```python
from build123d import *

# Parameters (mm, degrees)
F1_DEPTH = 30
F2_W     = 56
F2_H     = 56
F3_DEPTH = 100.001
F4_W     = 50
F4_H     = 15
F5_DEPTH = 60
F6_W     = 50
F6_H     = 15
F7_DEPTH = 30
F8_W     = 80
F8_H     = 80
F9_DEPTH = 2
F10_R    = 1
F11_R    = 1
F12_R    = 1
F13_R    = 1
F14_R    = 0.5
F15_R    = 0.5
F16_R    = 0.5


with BuildPart() as f1:
    # F0 (on Front) → F1 (new body, symmetric)
    with BuildSketch(Plane.XZ):
        Polygon((30, 49.2234811187), (0, 49.2234811187), (-30, 49.2234811187), (-30, -50.7765188813), (0, -21.0795458406), (30, -50.7765188813), align=None)
    extrude(amount=F1_DEPTH, both=True)

    # F2 (on face) → F3 (cut, through all)
    with BuildSketch(Plane.XY.offset(49.2234811187)):
        with Locations((-2.794e-06, 0)):
            Rectangle(F2_W, F2_H)
    extrude(amount=-F3_DEPTH, mode=Mode.SUBTRACT)

    # F4 (on face) → F5 (cut)
    with BuildSketch(Plane.XZ.offset(30)):
        with Locations((0, 38.2234811187)):
            Rectangle(F4_W, F4_H)
    extrude(amount=-F5_DEPTH, mode=Mode.SUBTRACT)

    # F6 (on Right) → F7 (cut, symmetric)
    with BuildSketch(Plane.YZ):
        with Locations((0, 38.2234811187)):
            Rectangle(F6_W, F6_H)
    extrude(amount=F7_DEPTH, both=True, mode=Mode.SUBTRACT)

    # F8 (on face) → F9 (join)
    with BuildSketch(Plane.XY.offset(49.2234811187)):
        Rectangle(F8_W, F8_H)
    extrude(amount=-F9_DEPTH)

    # F10
    f10_edges = [f1.edges().sort_by_distance(p)[0] for p in [
        (-29.000001, 25, 30.723481),
        (-29.000001, -25, 30.723481),
        (-29.000001, -25, 45.723481),
        (-29.000001, 25, 45.723481),
    ]]
    fillet(f10_edges, radius=F10_R)

    # F11
    f11_edges = [f1.edges().sort_by_distance(p)[0] for p in [
        (-25, 29, 45.723481),
        (-25, 29, 30.723481),
        (25, 29, 30.723481),
        (25, 29, 45.723481),
    ]]
    fillet(f11_edges, radius=F11_R)

    # F12
    f12_edges = [f1.edges().sort_by_distance(p)[0] for p in [
        (28.999999, 25, 45.723481),
        (28.999999, -25, 45.723481),
        (28.999999, -25, 30.723481),
        (28.999999, 25, 30.723481),
    ]]
    fillet(f12_edges, radius=F12_R)

    # F13
    f13_edges = [f1.edges().sort_by_distance(p)[0] for p in [
        (25, -29, 30.723481),
        (25, -29, 45.723481),
        (-25, -29, 45.723481),
        (-25, -29, 30.723481),
    ]]
    fillet(f13_edges, radius=F13_R)

    # F14
    f14_edges = [f1.edges().sort_by_distance(p)[0] for p in [
        (30, 30, -1.776519),
        (30, -30, -1.776519),
        (-30, 30, -1.776519),
        (-30, -30, -1.776519),
    ]]
    fillet(f14_edges, radius=F14_R)

    # F15
    f15_edges = [f1.edges().sort_by_distance(p)[0] for p in [
        (40, -40, 48.223481),
        (40, 0, 49.223481),
        (40, 0, 47.223481),
        (0, -40, 47.223481),
        (0, -40, 49.223481),
        (-40, -40, 48.223481),
        (-40, 0, 47.223481),
        (-40, 0, 49.223481),
        (0, 40, 47.223481),
        (0, 40, 49.223481),
        (-40, 40, 48.223481),
        (40, 40, 48.223481),
    ]]
    fillet(f15_edges, radius=F15_R)

    # F16
    f16_edges = [f1.edges().sort_by_distance(p)[0] for p in [
        (0, 30, 47.223481),
    ]]
    fillet(f16_edges, radius=F16_R)


solid = f1.part
```
Here's how the part is built. I have some questions about the finished solid (model axes, mm). A direction names the side the tool comes from. Coordinates: 2 decimals unless noted, no trailing zeros. Write each loop counter-clockwise with the first axis right and the second up, starting at its lowest first coordinate (ties: lowest second). Pieces come first, ordered by that corner, then holes. Notation, with made-up numbers: (87.5, 82.5) - (130.5, 82.5) arc R21 ccw to (130.5, 91.5) - close; hole circle Ø9 at (37, 50.5). An arc over 180 degrees is marked (long way). One line per item, written item: value.
1) On a 3-axis mill with a long thin cutter (end or side, diameter ignored), from which of +Z, -Z, +X, -X, +Y, -Y can I reach the whole of each face in a straight line? I mean faces 5 (the flat face through (28.263, -0.14, -49.057)), 6 (the flat face through (-1, 1, 49.223)), 7 (the flat face through (0, -30, -1)), 8 (the flat face through (0, 0, 47.223)), 9 (the flat face through (-30, 0, -12)). Say none if no direction works.
Model answer:
face 5: -Z, +Y, -Y
face 6: +Z, +X, -X, +Y, -Y
face 7: -Z, +X, -X, -Y
face 8: -Z
face 9: -Z, -X, +Y, -Y
2) Suppose I cut it at D-D on z = 38. Write out the boundary of the cut face in (x, y).
Model answer:
outline: (-30, -29.5) arc R0.5 ccw to (-29.5, -30) - (-25, -30) - (-25, -28) - (-28, -28) - (-28, -25) - (-30, -25) - close; (-30, 25) - (-28, 25) - (-28, 28) - (-25, 28) - (-25, 30) - (-29.5, 30) arc R0.5 ccw to (-30, 29.5) - close; (25, -30) - (29.5, -30) arc R0.5 ccw to (30, -29.5) - (30, -25) - (28, -25) - (28, -28) - (25, -28) - close; (25, 28) - (28, 28) - (28, 25) - (30, 25) - (30, 29.5) arc R0.5 ccw to (29.5, 30) - (25, 30) - close
3) Suppose I cut it at C-C on x = -22. Write out the boundary of the cut face in (y, z).
Model answer:
outline: (-40, 47.72) arc R0.5 ccw to (-39.5, 47.22) - (-30.5, 47.22) arc R0.5 cw to (-30, 46.72) - (-30, 45.72) - (-28, 45.72) - (-28, 47.22) - (28, 47.22) - (28, 45.72) - (30, 45.72) - (30, 46.72) arc R0.5 cw to (30.5, 47.22) - (39.5, 47.22) arc R0.5 ccw to (40, 47.72) - (40, 48.72) arc R0.5 ccw to (39.5, 49.22) - (-39.5, 49.22) arc R0.5 ccw to (-40, 48.72) - close; (-30, -42.86) - (-28, -42.86) - (-28, 30.72) - (-30, 30.72) - close; (28, -42.86) - (30, -42.86) - (30, 30.72) - (28, 30.72) - close
4) Suppose I cut it at A-A on z = 23. Write out the boundary of the cut face in (x, y).
Model answer:
outline: (-30, -29.5) arc R0.5 ccw to (-29.5, -30) - (29.5, -30) arc R0.5 ccw to (30, -29.5) - (30, 29.5) arc R0.5 ccw to (29.5, 30) - (-29.5, 30) arc R0.5 ccw to (-30, 29.5) - close; hole (-28, -28) - (28, -28) - (28, 28) - (-28, 28) - close
5) I'm going to push flat-ended pins straight in: P1, Ø17, axis at x = 8, z = -0.5, coming from the +Y side; P2, Ø1, axis at y = 29, z = 41, coming from the -X side; P3, Ø1, axis at y = 29.5, z = 41, coming from the +X side; P4, Ø1, axis at y = -31.5, z = 1.5, coming from the +X side. Where does each tip first touch, or does it pass through?
Model answer:
P1: stops at y = 30
P2: stops at x = -30
P3: stops at x = 30
P4: passes through
6) We'd pull the mould along X, two halves only. Please class faces 1 (the flat face through (0, 28, 0)), 2 (the flat face through (28, 0, -11)), 3 (the flat face through (30, 0, -3)), 4 (the flat face through (0, 30, -1)): pulls with the +X half, pulls with the -X half, needs draft (parallel to the pull), parting line crosses it, or undercut.
Model answer:
face 1: undercut
face 2: undercut
face 3: pulls with the +X half
face 4: needs draft
7) I need wall thicknesses on line 1 along X through (y, z) = (-21, -12); line 2 along Z through (x, y) = (4.5, 18.5). Which ranges of each line are inside material? Lowest first, please.
Model answer:
line 1: x = -30 to -28, 28 to 30
line 2: z = 47.22 to 49.22
8) Suppose I cut it at B-B on y = -19. Write out the boundary of the cut face in (x, z).
Model answer:
outline: (-40, 47.72) arc R0.5 ccw to (-39.5, 47.22) - (-30.5, 47.22) arc R0.5 cw to (-30, 46.72) - (-30, 45.72) - (-28, 45.72) - (-28, 47.22) - (28, 47.22) - (28, 45.72) - (30, 45.72) - (30, 46.72) arc R0.5 cw to (30.5, 47.22) - (39.5, 47.22) arc R0.5 ccw to (40, 47.72) - (40, 48.72) arc R0.5 ccw to (39.5, 49.22) - (-39.5, 49.22) arc R0.5 ccw to (-40, 48.72) - close; (-30, -50.78) - (-28, -48.8) - (-28, 30.72) - (-30, 30.72) - close; (28, -48.8) - (30, -50.78) - (30, 30.72) - (28, 30.72) - close
